Work out the finished part from the listing and answer in its coordinate system (mm). Face numbers are marked on the shaded views. Round coordinates to 2 decimals unless told otherwise and drop trailing zeros. Write each loop counter-clockwise with the first axis right and the second up, starting at its lowest first coordinate (ties: lowest second). Pieces come first, ordered by that corner, then holes.
from build123d import *

# Parameters (mm, degrees)
SKETCH1_R           = 1.85
BOSS_EXTRUDE1_DEPTH = 2.05
CHAMFER1_SIZE       = 0.25


with BuildPart() as part:
    # Sketch1 → Boss-Extrude1 (new body)
    with BuildSketch(Plane(origin=(0, 0, 0), x_dir=(1, 0, 0), z_dir=(0, 1, 0))):
        with BuildLine():
            Line((-2.1375, 3.1375), (2.1375, 3.1375))
            ThreePointArc((2.1375, 3.1375), (2.844606781, 2.844606781), (3.1375, 2.1375))
            Line((3.1375, 2.1375), (3.1375, -2.1375))
            ThreePointArc((3.1375, -2.1375), (2.844606781, -2.844606781), (2.1375, -3.1375))
            Line((2.1375, -3.1375), (-2.1375, -3.1375))
            ThreePointArc((-2.1375, -3.1375), (-2.844606781, -2.844606781), (-3.1375, -2.1375))
            Line((-3.1375, -2.1375), (-3.1375, 2.1375))
            ThreePointArc((-3.1375, 2.1375), (-2.844606781, 2.844606781), (-2.1375, 3.1375))
        make_face()
        with Locations(Location((0, 0, 0), (0, 0, 270))):
            Circle(SKETCH1_R, mode=Mode.SUBTRACT)
    extrude(amount=BOSS_EXTRUDE1_DEPTH)

    # Chamfer1
    chamfer1_edges = [part.edges().sort_by_distance(p)[0] for p in [
        (2.844606781, 2.05, -2.844606781),
        (3.1375, 0, 0),
        (2.844606781, 0, 2.844606781),
        (0, 2.05, -3.1375),
        (-2.844606781, 2.05, -2.844606781),
        (-3.1375, 2.05, 0),
        (-2.844606781, 2.05, 2.844606781),
        (0, 2.05, 3.1375),
        (2.844606781, 2.05, 2.844606781),
        (3.1375, 2.05, 0),
        (0, 0, 3.1375),
        (-2.844606781, 0, 2.844606781),
        (-3.1375, 0, 0),
        (-2.844606781, 0, -2.844606781),
        (0, 0, -3.1375),
        (2.844606781, 0, -2.844606781),
    ]]
    chamfer(chamfer1_edges, length=CHAMFER1_SIZE)


solid = part.part
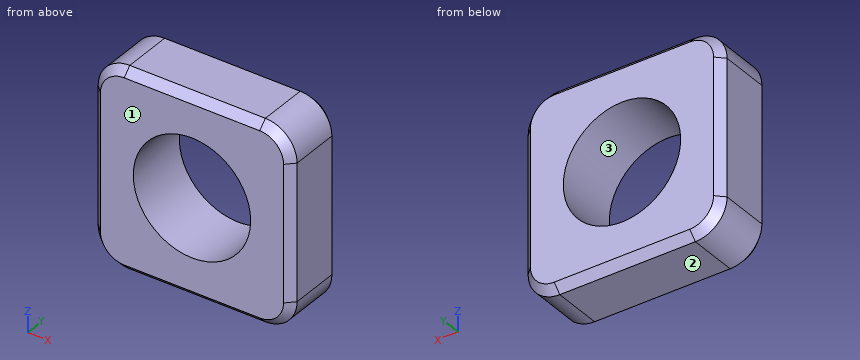
Q1. Find section B-B (x = 0). Determine the outline of the cut face in (y, z).
Q2. The mould has two halves that part along Z. Classify the marked faces 1, 2 and 3: +Z half, -Z half, draft (parallel to the pull), parting line (faces both ways), or undercut.
Q3. Find section C-C (y = 1). Determine the outline of the cut face in (x, z).
Q4. Find section A-A (z = -1.75). Determine the outline of the cut face in (x, y), plus the area to 3 significant figures.
Q5. Find section D-D (y = 1.9). Determine the outline of the cut face in (x, z).
Q6. Find the intervals of material crossed by L1, parallel to X at y = 1.55, z = 0; L2, parallel to Z at x = 0.5, y = 1.6; L3, parallel to X at y = 0.75, z = -0.75, in increasing order.
Report:
1. outline: (0, -2.89) - (0.25, -3.14) - (1.8, -3.14) - (2.05, -2.89) - (2.05, -1.85) - (0, -1.85) - close; (0, 1.85) - (2.05, 1.85) - (2.05, 2.89) - (1.8, 3.14) - (0.25, 3.14) - (0, 2.89) - close
2. face 1: draft
2. face 2: -Z half
2. face 3: undercut
3. outline: (-3.14, -2.14) arc R1 ccw to (-2.14, -3.14) - (2.14, -3.14) arc R1 ccw to (3.14, -2.14) - (3.14, 2.14) arc R1 ccw to (2.14, 3.14) - (-2.14, 3.14) arc R1 ccw to (-3.14, 2.14) - close; hole circle Ø3.7 at (0, 0)
4. outline: (-3.14, 0.25) - (-2.89, 0) - (-0.6, 0) - (-0.6, 2.05) - (-2.89, 2.05) - (-3.14, 1.8) - close; (0.6, 0) - (2.89, 0) - (3.14, 0.25) - (3.14, 1.8) - (2.89, 2.05) - (0.6, 2.05) - close
4. area: 10.3 mm2
5. outline: (-3.04, -2.14) arc R0.9 ccw to (-2.14, -3.04) - (2.14, -3.04) arc R0.9 ccw to (3.04, -2.14) - (3.04, 2.14) arc R0.9 ccw to (2.14, 3.04) - (-2.14, 3.04) arc R0.9 ccw to (-3.04, 2.14) - close; hole circle Ø3.7 at (0, 0)
6. L1: x = -3.14 to -1.85, 1.85 to 3.14
6. L2: z = -3.14 to -1.78, 1.78 to 3.14
6. L3: x = -3.14 to -1.69, 1.69 to 3.14
